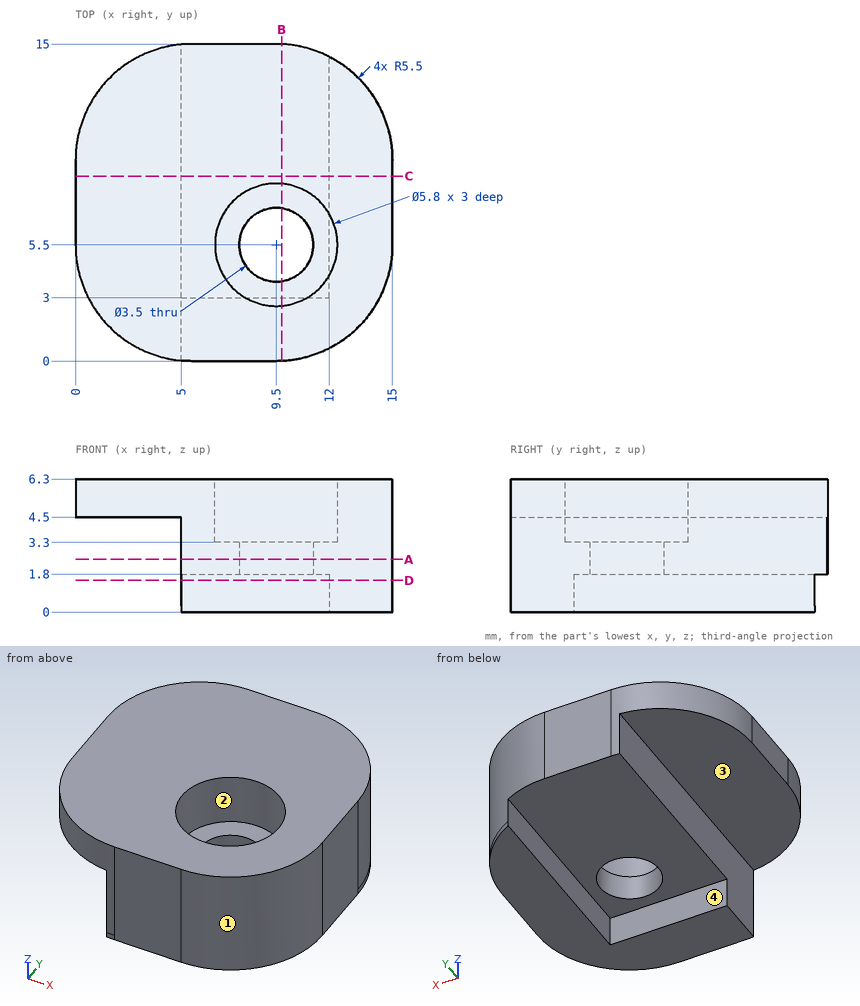
Here's the drawing with two shaded views (mm, measured from the low corner). I have some questions. A direction names the side the tool comes from. Coordinates: 2 decimals unless noted, no trailing zeros. Loops run counter-clockwise (first coordinate to the right, second up) from the corner with the lowest first, then second, coordinate; pieces in that order, holes last. Notation, with made-up numbers: M -3.5,4 L 32.5,4 A15 ccw 32.5,18 Z; hole C -0.75,40 d1. An arc over 180 degrees is marked long. Put each result on its own line as item: value. Start each with the question number.
(1) Imagine slicing it at C-C on y = 8.75. List the corners of the cut face in (x, z) for me.
(2) Imagine slicing it at D-D on z = 1.5. List the corners of the cut face in (x, y) for me, and give its area (3 significant figures).
(3) Imagine slicing it at B-B on x = 9.75. List the corners of the cut face in (y, z) for me, and give its area (3 significant figures).
(4) Imagine slicing it at A-A on z = 2.5. List the corners of the cut face in (x, y) for me, and give its area (3 significant figures).
(5) Will these pins go through, and if not, where does the flat tip stop? pin 1 Ø5.5 at (x, y) = (9.5, 5.5) entering from +Z; pin 2 Ø2 at (y, z) = (5, 1.5) entering from -X; pin 3 Ø1.4 at (y, z) = (11, 0.5) entering from -X; pin 4 Ø0.9 at (x, z) = (7.5, 1.5) entering from +Y.
(6) I need wall thicknesses on probe 1 along Y at (x, z) = (9.5, 4.15); probe 2 along Z at (x, y) = (11, 11.5); probe 3 along Z at (x, y) = (2.5, 6.5). Which ranges of each line are inside material? Lowest first, please.
(7) Which directions (+Z, -Z, +X, -X, +Y, -Y) give clear straight access to the entire face, cutting with the end or side of a thin tool? Please do the marked faces 1, 2, 3 and 4.
Worked answers:
1. outline: M 0,4.5 L 5,4.5 L 5,1.8 L 12,1.8 L 12,0 L 15,0 L 15,6.3 L 0,6.3 Z
2. outline: M 5,0.02 A5.5 ccw 5.5,0 L 9.5,0 A5.5 ccw 15,5.5 L 15,9.5 A5.5 ccw 12,14.4 L 12,3 L 5,3 Z
2. area: 53.5 mm2
3. outline: M 0.01,0 L 3,0 L 3,1.8 L 3.77,1.8 L 3.77,3.3 L 2.61,3.3 L 2.61,6.3 L 0.01,6.3 Z; M 7.23,1.8 L 14.99,1.8 L 14.99,6.3 L 8.39,6.3 L 8.39,3.3 L 7.23,3.3 Z
3. area: 50.3 mm2
4. outline: M 5,0.02 A5.5 ccw 5.5,0 L 9.5,0 A5.5 ccw 15,5.5 L 15,9.5 A5.5 ccw 9.5,15 L 5.5,15 A5.5 ccw 5,14.98 Z; hole C 9.5,5.5 d3.5
4. area: 127 mm2
5. pin 1: stops at z = 3.3
5. pin 2: stops at x = 5
5. pin 3: stops at x = 12
5. pin 4: stops at y = 15
6. probe 1: y = 0 to 2.6, 8.4 to 15
6. probe 2: z = 1.8 to 6.3
6. probe 3: z = 4.5 to 6.3
7. face 1: +Z, -Z, +X, -Y
7. face 2: +Z
7. face 3: -Z, -X, +Y, -Y
7. face 4: -Z, -X, +Y
